The drawing under review shows one solid part. Ordinate dimensions are in mm from its lowest x, y, z. A direction names the side the tool comes from. Round coordinates to 2 decimals unless told otherwise and drop trailing zeros. Order: outer loops, then holes, each group sorted by start corner. A loop starts at its lowest first (then second) coordinate and runs counter-clockwise, first axis right, second up. Notation, with made-up numbers: M -3.5,9.5 L 48.5,9.5 A14 ccw 48.5,24.5 Z; hole C -23.5,28.25 d9. An arc over 180 degrees is marked long. Answer as a JSON object with one key per item and string values.
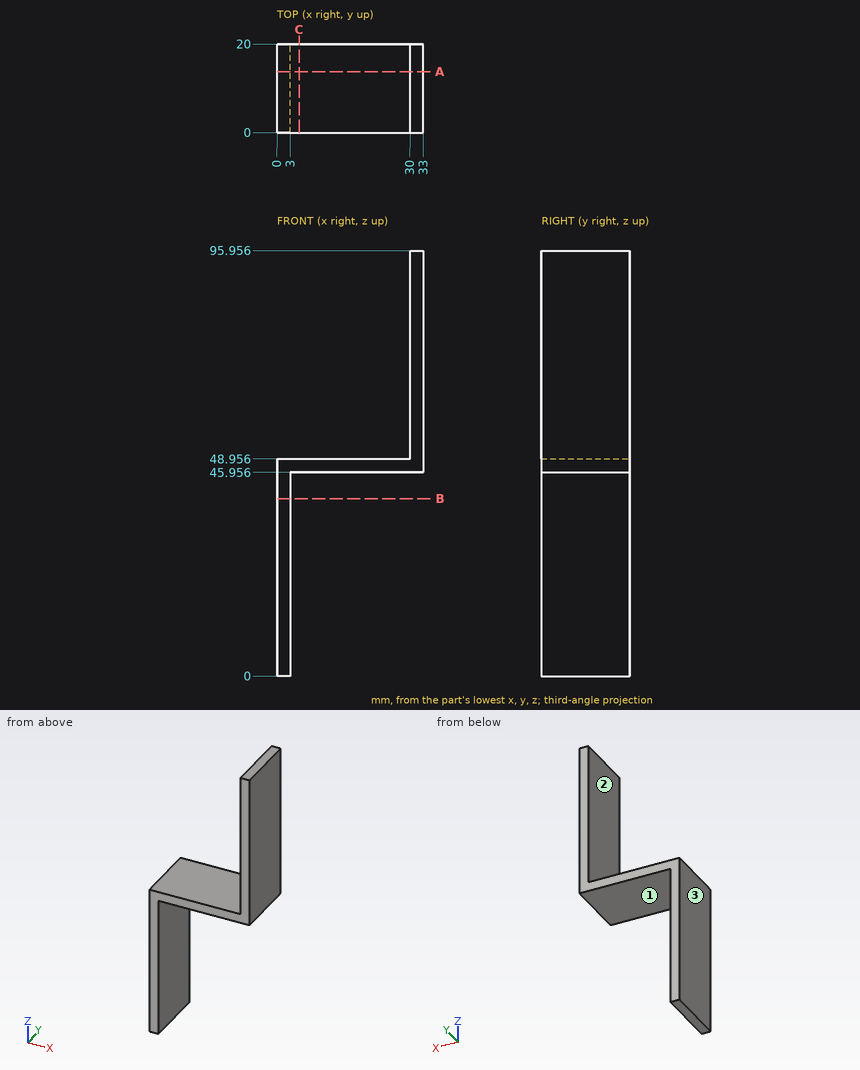
1) Add section B-B on z = 40. State the section outline as (x, y) points.
Geometry check:
{"outline": "M 0,0 L 3,0 L 3,20 L 0,20 Z"}
2) Insertion check: P1, Ø10, axis at x = 21, y = 8.5, coming from the -Z side; P2, Ø12, axis at x = 8, y = 12, coming from the +Z side; P3, Ø6, axis at y = 11, z = 13, coming from the +X side; P4, Ø4, axis at x = 3.5, z = 22.5, coming from the -Y side. Each pin has a flat end and moves straight along its axis. Give the tip position at first contact, or say it passes through.
Geometry check:
{"P1": "stops at z = 45.96", "P2": "stops at z = 48.96", "P3": "stops at x = 3", "P4": "stops at y = 0"}
3) Add section A-A on y = 13.75. State the section outline as (x, z) points, and give its area (3 significant figures).
Geometry check:
{"outline": "M 0,0 L 3,0 L 3,45.96 L 33,45.96 L 33,95.96 L 30,95.96 L 30,48.96 L 0,48.96 Z", "area": "378 mm²"}
4) For L1, parallel to Z at x = 14, y = 5.5; L2, parallel to X at y = 9.75, z = 17.5; L3, parallel to X at y = 16.5, z = 55, list the stretches that pass through material, from the lowest coordinate up.
Geometry check:
{"L1": "z = 45.96 to 48.96", "L2": "x = 0 to 3", "L3": "x = 30 to 33"}
5) Machinability: for the marked faces 1, 2 and 3, which of the approach directions +Z, -Z, +X, -X, +Y, -Y give a long, thin tool a straight path to every point of the face, cutting with its end or side? Answer none if there is none.
Geometry check:
{"face 1": "-Z, +X, +Y, -Y", "face 2": "+Z, -X, +Y, -Y", "face 3": "+Z, -Z, -X, +Y, -Y"}
6) Add section C-C on x = 5. State the section outline as (y, z) points, and give its area (3 significant figures).
Geometry check:
{"outline": "M 0,45.96 L 20,45.96 L 20,48.96 L 0,48.96 Z", "area": "60.0 mm²"}
